```python
from build123d import *

# Parameters (mm, degrees)
F1_DEPTH = 13.3
F3_DEPTH = 7.3


with BuildPart() as f1:
    # F0 (on Top) → F1 (new body)
    with BuildSketch(Plane.XY):
        with BuildLine():
            Line((35.104722, 81.694619), (-28.895278, 81.694619))
            ThreePointArc((-28.895278, 81.694619), (-35.966346, 78.765687), (-38.895278, 71.694619))
            Line((-38.895278, 71.694619), (-38.895278, -72.305381))
            ThreePointArc((-38.895278, -72.305381), (-35.966346, -79.376448), (-28.895278, -82.305381))
            Line((-28.895278, -82.305381), (35.104722, -82.305381))
            ThreePointArc((35.104722, -82.305381), (42.17579, -79.376448), (45.104722, -72.305381))
            Line((45.104722, -72.305381), (45.104722, 71.694619))
            ThreePointArc((45.104722, 71.694619), (42.17579, 78.765687), (35.104722, 81.694619))
        make_face()
    extrude(amount=F1_DEPTH)

    # F2 (on Top) → F3 (cut)
    with BuildSketch(Plane.XY):
        with BuildLine():
            Line((32.104722, 78.694619), (-25.895278, 78.694619))
            ThreePointArc((-25.895278, 78.694619), (-32.966346, 75.765687), (-35.895278, 68.694619))
            Line((-35.895278, 68.694619), (-35.895278, -69.305381))
            ThreePointArc((-35.895278, -69.305381), (-32.966346, -76.376448), (-25.895278, -79.305381))
            Line((-25.895278, -79.305381), (32.104722, -79.305381))
            ThreePointArc((32.104722, -79.305381), (39.17579, -76.376448), (42.104722, -69.305381))
            Line((42.104722, -69.305381), (42.104722, 68.694619))
            ThreePointArc((42.104722, 68.694619), (39.17579, 75.765687), (32.104722, 78.694619))
        make_face()
    extrude(amount=F3_DEPTH, mode=Mode.SUBTRACT)


solid = f1.part
```
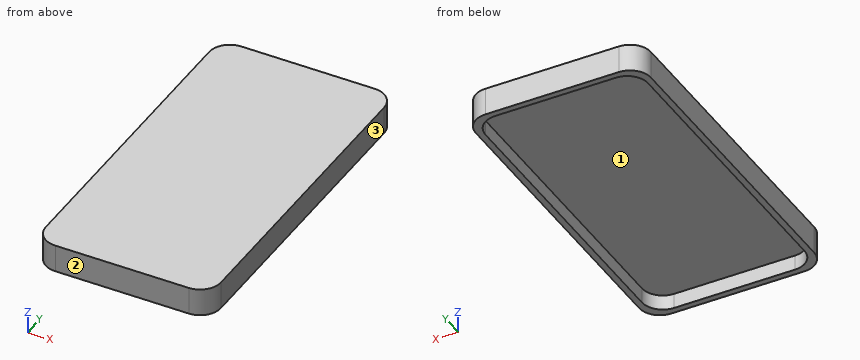
Geometry check sheet. Reference: the model listing, model coordinates, mm. Face numbers are marked on the shaded views. Give positions to 0.01 mm unless a question says otherwise; leave off trailing zeros. Loops run counter-clockwise (first coordinate to the right, second up) from the corner with the lowest first, then second, coordinate; pieces in that order, holes last. Notation, with made-up numbers: M -12.5,-1.75 L 46.5,-1.75 A18 ccw 46.5,27.25 Z; hole C 76,-37.5 d3. An arc over 180 degrees is marked long. Write item = value, one per line.
(1) Release check for a two-part mould opening along X. For the marked faces 1, 2 and 3 record: released by +X, released by -X, zero draft, split by the parting line, or undercut.
Answer below:
face_1 = undercut
face_2 = zero draft
face_3 = released by +X
(2) Sectioned sample at B-B, the plane y = -22.5. Record the cut outline in (x, z), plus the area to 3 significant figures.
Answer below:
outline = M -38.9,0 L -35.9,0 L -35.9,7.3 L 42.1,7.3 L 42.1,0 L 45.1,0 L 45.1,13.3 L -38.9,13.3 Z
area = 548 mm2
(3) Sectioned sample at A-A, the plane z = 2. Record the cut outline in (x, y).
Answer below:
outline = M -38.9,-72.31 A10 ccw -28.9,-82.31 L 35.1,-82.31 A10 ccw 45.1,-72.31 L 45.1,71.69 A10 ccw 35.1,81.69 L -28.9,81.69 A10 ccw -38.9,71.69 Z; hole M -35.9,-69.31 A10 ccw -25.9,-79.31 L 32.1,-79.31 A10 ccw 42.1,-69.31 L 42.1,68.69 A10 ccw 32.1,78.69 L -25.9,78.69 A10 ccw -35.9,68.69 Z
(4) Material ranges on line 1 (X direction, y = 18.5, z = 6.25); line 2 (Y direction, x = -18.5, z = 4.75); line 3 (Z direction, x = -26, y = -26), recorded low to high. Write a range as [from, to].
Answer below:
line_1 = [-38.9, -35.9], [42.1, 45.1]
line_2 = [-82.31, -79.31], [78.69, 81.69]
line_3 = [7.3, 13.3]
(5) Gauge pin test, flat end, axial feed: pin 1 Ø23.5 at (x, y) = (15, -3) entering from -Z. Record the tip position at first contact, or that the pin passes through.
Answer below:
pin_1 = 7.3
(6) Sectioned sample at C-C, the plane x = -13.5. Record the cut outline in (y, z).
Answer below:
outline = M -82.31,0 L -79.31,0 L -79.31,7.3 L 78.69,7.3 L 78.69,0 L 81.69,0 L 81.69,13.3 L -82.31,13.3 Z
